Geometry check sheet. Reference: the model listing, model coordinates, mm. Face numbers are marked on the shaded views. Round coordinates to 2 decimals unless told otherwise and drop trailing zeros. Order: outer loops, then holes, each group sorted by start corner. A loop starts at its lowest first (then second) coordinate and runs counter-clockwise, first axis right, second up. Notation, with made-up numbers: (-20.5, 52.25) -> (38.5, 52.25) arc R3 cw to (38.5, 57.25) -> close; hole circle Ø1 at (-35, 1). An arc over 180 degrees is marked (long way). Use a Markdown table: item, result. Add a question column.
Item 1: Mould release check, pull along Y, two halves, no side actions. Record for the marked faces 1, 2 and 3: pulls with the +Y half, pulls with the -Y half, needs draft (parallel to the pull), parting line crosses it, or undercut.
Item 2: Gauge pin test, flat ends, axial feed: pin 1 Ø1 at (x, z) = (18, 52.5) entering from +Y; pin 2 Ø3 at (y, z) = (-18.5, 59.5) entering from +X; pin 3 Ø1 at (x, z) = (4, 52.5) entering from +Y. Record the tip position at first contact, or that the pin passes through.
Item 3: Material ranges on probe 1 along Z at (x, y) = (10.25, 17.25); probe 2 along Z at (x, y) = (13.25, -17); probe 3 along Y at (x, z) = (2.65, 59.5), recorded low to high. Write a range as [from, to].
Item 4: Sectioned sample at B-B, the plane z = 61. Record the cut outline in (x, y) (3 decimals).
Item 5: Sectioned sample at D-D, the plane y = 0. Record the cut outline in (x, z), and give its area (3 significant figures).
Item 6: Sectioned sample at C-C, the plane z = 51. Record the cut outline in (x, y) (3 decimals), and give its area (3 significant figures).
Item 7: Sectioned sample at A-A, the plane y = -15.5. Record the cut outline in (x, z).
from build123d import *

# Parameters (mm, degrees)
F1_DEPTH = 79
F2_R     = 2.6
F3_DEPTH = 25.001
F6_DEPTH = 25
F7_W     = 6
F7_H     = 6
F8_DEPTH = 79.0010001


with BuildPart() as f1:
    # F0 (on Top) → F1 (new body)
    with BuildSketch(Plane.XY):
        with BuildLine():
            Line((0.5, -9.4868329805), (0.5, -24.9949994999))
            ThreePointArc((0.5, -24.9949994999), (25, 0), (0.5, 24.9949994999))
            Line((0.5, 24.9949994999), (0.5, 9.4868329805))
            ThreePointArc((0.5, 9.4868329805), (9.5, 0), (0.5, -9.4868329805))
        make_face()
    extrude(amount=F1_DEPTH)

    # F2 (on Right) → F3 (cut, through all)
    with BuildSketch(Plane.YZ):
        with Locations((-17.25, 19.5)):
            Circle(F2_R)
        with Locations((-17.25, 59.5)):
            Circle(F2_R)
        with Locations((17.25, 59.5)):
            Circle(F2_R)
        with Locations((17.25, 19.5)):
            Circle(F2_R)
    extrude(amount=F3_DEPTH, mode=Mode.SUBTRACT)

    # F5 (on offset) → F6 (cut)
    with BuildSketch(Plane(origin=(6.5, 0, 0), x_dir=(0, -1, 0), z_dir=(-1, 0, 0))):
        with BuildLine():
            ThreePointArc((12, 59.5), (17.25, 54.25), (22.5, 59.5))
            ThreePointArc((22.5, 59.5), (17.25, 64.75), (12, 59.5))
        make_face()
        with BuildLine():
            ThreePointArc((-12, 19.5), (-13.5376893988, 23.2123106012), (-17.25, 24.75))
            ThreePointArc((-17.25, 24.75), (-20.9623106012, 15.7876893988), (-12, 19.5))
        make_face()
    extrude(amount=-F6_DEPTH, mode=Mode.SUBTRACT)

    # F7 (on Top) → F8 (cut, through all)
    with BuildSketch(Plane.XY):
        with Locations((9, 0)):
            Rectangle(F7_W, F7_H)
    extrude(amount=F8_DEPTH, mode=Mode.SUBTRACT)


solid = f1.part
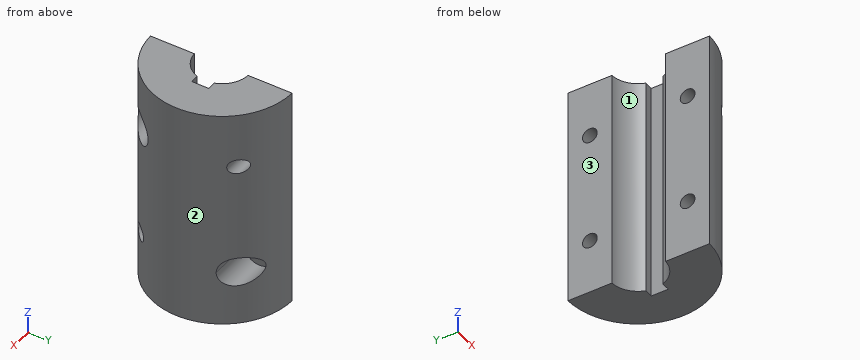
Found:
| question | item | result |
|---|---|---|
| 1 | face 1 | undercut |
| 1 | face 2 | parting line crosses it |
| 1 | face 3 | needs draft |
| 2 | pin 1 | stops at y = 17.85 |
| 2 | pin 2 | stops at x = 6.5 |
| 2 | pin 3 | stops at y = 24.75 |
| 3 | probe 1 | z = [0, 14.25], [24.75, 56.9], [62.1, 79] |
| 3 | probe 2 | z = [0, 16.91], [22.09, 54.26], [64.74, 79] |
| 3 | probe 3 | y = [-24.86, -19.85], [-14.65, -9.12], [9.12, 14.65], [19.85, 24.86] |
| 4 | outline | (0.5, -24.995) arc R25 ccw to (11.338, -22.281) -> (6.5, -22.281) -> (6.5, -19.374) -> (0.5, -19.374) -> close; (0.5, -15.126) -> (6.5, -15.126) -> (6.5, -12.219) -> (21.811, -12.219) arc R25 ccw to (19.905, 15.126) -> (0.5, 15.126) -> (0.5, 9.487) arc R9.5 cw to (9.014, 3) -> (12, 3) -> (12, -3) -> (9.014, -3) arc R9.5 cw to (0.5, -9.487) -> close; (0.5, 19.374) -> (15.801, 19.374) arc R25 ccw to (0.5, 24.995) -> close |
| 5 | outline | (12, 0) -> (25, 0) -> (25, 79) -> (12, 79) -> close |
| 5 | area | 1,030 mm2 |
| 6 | outline | (0.5, -24.995) arc R25 ccw to (0.5, 24.995) -> (0.5, 9.487) arc R9.5 cw to (9.014, 3) -> (12, 3) -> (12, -3) -> (9.014, -3) arc R9.5 cw to (0.5, -9.487) -> close |
| 6 | area | 809 mm2 |
| 7 | outline | (0.5, 0) -> (19.62, 0) -> (19.62, 17.58) -> (0.5, 17.58) -> close; (0.5, 21.42) -> (19.62, 21.42) -> (19.62, 54.55) -> (6.5, 54.55) -> (6.5, 57.58) -> (0.5, 57.58) -> close; (0.5, 61.42) -> (6.5, 61.42) -> (6.5, 64.45) -> (19.62, 64.45) -> (19.62, 79) -> (0.5, 79) -> close |
